```python
from build123d import *

# Parameters (mm, degrees)
F0_W         = 62.5
F0_H         = 36.5
F0_W_2       = 58.5
F0_H_2       = 31.5
F1_DEPTH     = 7
F3_DEPTH     = 1.5
F4_W         = 62.5
F4_H         = 36.5
F5_DEPTH     = 3
F7_DEPTH     = 2.5
F8_R         = 2.5
F9_T1_DEPTH  = 57.5
F9_T3_DEPTH  = 31.5
F9_T6_ANGLE  = 90
F9_T8_ANGLE  = 90
F9_T10_ANGLE = 90
F9_T12_ANGLE = 90
F10_W        = 1.25
F10_H        = 8.5
F11_DEPTH    = 2
F13_DEPTH    = 3


# Not quite as in the source:
# - a fillet or chamfer that OpenCascade refuses, or shapes differently, is made with other operations: its cross-section is extruded or revolved along the edge and cut away or added
# - a feature names something its author has since deleted; it is built from what else it names


with BuildPart() as f1:
    # F0 (on Top) → F1 (new body)
    with BuildSketch(Plane.XY):
        with Locations((0.5, 0.5)):
            Rectangle(F0_W, F0_H)
        with Locations((1, 0.5)):
            Rectangle(F0_W_2, F0_H_2, mode=Mode.SUBTRACT)
    extrude(amount=F1_DEPTH)

    # F2 (on face) → F3 (join)
    with BuildSketch(Plane.XY.offset(7)):
        Polygon((30.25, 16.25), (-28.25, 16.25), (-28.25, -15.25), (30.25, -15.25), (30.25, -6), (30.25, 7), align=None)
    extrude(amount=-F3_DEPTH)

    # F4 (on face) → F5 (join)
    with BuildSketch(Plane(origin=(0, 0, 0), x_dir=(1, 0, 0), z_dir=(0, 0, -1))):
        with Locations((0.5, -0.5)):
            Rectangle(F4_W, F4_H)
        Polygon((-29.5, -17.522141248), (-29.5, 16.5), (30.25, 16.5), (30.25, 15.25), (30.25, -16.25), (30.25, -17.522141248), align=None, mode=Mode.SUBTRACT)
    extrude(amount=F5_DEPTH)

    # F6 (on face) → F7 (cut)
    with BuildSketch(Plane.YZ.offset(-28.25)):
        with BuildLine():
            Line((4, 5.5), (-3, 5.5))
            ThreePointArc((-3, 5.5), (-3.5303300859, 5.2803300859), (-3.75, 4.75))
            Line((-3.75, 4.75), (-3.75, 3.5))
            ThreePointArc((-3.75, 3.5), (-3.1642135624, 2.0857864376), (-1.75, 1.5))
            Line((-1.75, 1.5), (2.75, 1.5))
            ThreePointArc((2.75, 1.5), (4.1642135624, 2.0857864376), (4.75, 3.5))
            Line((4.75, 3.5), (4.75, 4.75))
            ThreePointArc((4.75, 4.75), (4.5303300859, 5.2803300859), (4, 5.5))
        make_face()
    extrude(amount=-F7_DEPTH, mode=Mode.SUBTRACT)

    # F8
    f8_edges = [f1.edges().sort_by_distance(p)[0] for p in [
        (-30.75, 18.75, 2),
        (-30.75, -17.75, 2),
        (31.75, 18.75, 2),
        (31.75, -17.75, 2),
    ]]
    fillet(f8_edges, radius=F8_R)

    # F9: fillet of radius 2 on 8 edges, made by hand

    # F9_s2 → F9_t1 (cut)
    with BuildSketch(Plane.YZ.offset(-28.25)):
        with BuildLine():
            ThreePointArc((18.75, 5), (18.1642135624, 6.4142135624), (16.75, 7))
            Line((16.75, 7), (18.75, 7))
            Line((18.75, 7), (18.75, 5))
        make_face()
        with BuildLine():
            ThreePointArc((-15.75, 7), (-17.1642135624, 6.4142135624), (-17.75, 5))
            Line((-17.75, 5), (-17.75, 7))
            Line((-17.75, 7), (-15.75, 7))
        make_face()
    extrude(amount=F9_T1_DEPTH, mode=Mode.SUBTRACT)

    # F9_s4 → F9_t3 (cut)
    with BuildSketch(Plane.XZ.offset(-16.25)):
        with BuildLine():
            ThreePointArc((29.75, 7), (31.1642135624, 6.4142135624), (31.75, 5))
            Line((31.75, 5), (31.75, 7))
            Line((31.75, 7), (29.75, 7))
        make_face()
        with BuildLine():
            ThreePointArc((-28.75, 7), (-30.1642135624, 6.4142135624), (-30.75, 5))
            Line((-30.75, 5), (-30.75, 7))
            Line((-30.75, 7), (-28.75, 7))
        make_face()
    extrude(amount=F9_T3_DEPTH, mode=Mode.SUBTRACT)

    # F9_s5 → F9_t6 (revolve, cut)
    with BuildSketch(Plane.YZ.offset(29.25)):
        with BuildLine():
            ThreePointArc((16.75, 7), (18.1642135624, 6.4142135624), (18.75, 5))
            Line((18.75, 5), (18.75, 7))
            Line((18.75, 7), (16.75, 7))
        make_face()
    revolve(axis=Axis((29.25, 16.25, 7), (0, 0, -1)), revolution_arc=F9_T6_ANGLE, mode=Mode.SUBTRACT)

    # F9_s7 → F9_t8 (revolve, cut)
    with BuildSketch(Plane.YZ.offset(-28.25)):
        with BuildLine():
            ThreePointArc((16.75, 7), (18.1642135624, 6.4142135624), (18.75, 5))
            Line((18.75, 5), (18.75, 7))
            Line((18.75, 7), (16.75, 7))
        make_face()
    revolve(axis=Axis((-28.25, 16.25, 7), (0, 0, 1)), revolution_arc=F9_T8_ANGLE, mode=Mode.SUBTRACT)

    # F9_s9 → F9_t10 (revolve, cut)
    with BuildSketch(Plane.XZ.offset(15.25)):
        with BuildLine():
            ThreePointArc((29.75, 7), (31.1642135624, 6.4142135624), (31.75, 5))
            Line((31.75, 5), (31.75, 7))
            Line((31.75, 7), (29.75, 7))
        make_face()
    revolve(axis=Axis((29.25, -15.25, 7), (0, 0, -1)), revolution_arc=F9_T10_ANGLE, mode=Mode.SUBTRACT)

    # F9_s11 → F9_t12 (revolve, cut)
    with BuildSketch(Plane.XZ.offset(15.25)):
        with BuildLine():
            ThreePointArc((-28.75, 7), (-30.1642135624, 6.4142135624), (-30.75, 5))
            Line((-30.75, 5), (-30.75, 7))
            Line((-30.75, 7), (-28.75, 7))
        make_face()
    revolve(axis=Axis((-28.25, -15.25, 7), (0, 0, 1)), revolution_arc=F9_T12_ANGLE, mode=Mode.SUBTRACT)

    # F10 (on face) → F11 (cut)
    with BuildSketch(Plane(origin=(0, 0, 0), x_dir=(1, 0, 0), z_dir=(0, 0, -1))):
        with Locations((-28.875, -0.5)):
            Rectangle(F10_W, F10_H)
    extrude(amount=-F11_DEPTH, mode=Mode.SUBTRACT)

    # F12 (on face) → F13 (cut)
    with BuildSketch(Plane.XY.offset(7)):
        with BuildLine():
            ThreePointArc((22.6871086181, -10.5021475209), (24.4149310408, -5.3769082449), (25, 0))
            ThreePointArc((25, 0), (24.4149310408, 5.3769082449), (22.6871086181, 10.5021475209))
            Line((22.6871086181, 10.5021475209), (21.325882101, 9.8720186697))
            ThreePointArc((21.325882101, 9.8720186697), (22.9500351783, 5.0542937502), (23.5, 0))
            ThreePointArc((23.5, 0), (22.9500351783, -5.0542937502), (21.325882101, -9.8720186697))
            Line((21.325882101, -9.8720186697), (22.6871086181, -10.5021475209))
        make_face()
        with BuildLine():
            ThreePointArc((19.5109134115, -9.031846868), (20.9968406951, -4.6241410906), (21.5, 0))
            ThreePointArc((21.5, 0), (20.9968406951, 4.6241410906), (19.5109134115, 9.031846868))
            Line((19.5109134115, 9.031846868), (18.1496868945, 8.4017180168))
            ThreePointArc((18.1496868945, 8.4017180168), (19.5319448326, 4.3015265959), (20, 0))
            ThreePointArc((20, 0), (19.5319448326, -4.3015265959), (18.1496868945, -8.4017180168))
            Line((18.1496868945, -8.4017180168), (19.5109134115, -9.031846868))
        make_face()
        with BuildLine():
            ThreePointArc((16.334718205, -7.5615462151), (17.5787503494, -3.8713739363), (18, 0))
            ThreePointArc((18, 0), (17.5787503494, 3.8713739363), (16.334718205, 7.5615462151))
            Line((16.334718205, 7.5615462151), (14.9734916879, 6.9314173638))
            ThreePointArc((14.9734916879, 6.9314173638), (16.1138544869, 3.5487594416), (16.5, 0))
            ThreePointArc((16.5, 0), (16.1138544869, -3.5487594416), (14.9734916879, -6.9314173638))
            Line((14.9734916879, -6.9314173638), (16.334718205, -7.5615462151))
        make_face()
    extrude(amount=-F13_DEPTH, mode=Mode.SUBTRACT)


solid = f1.part
```
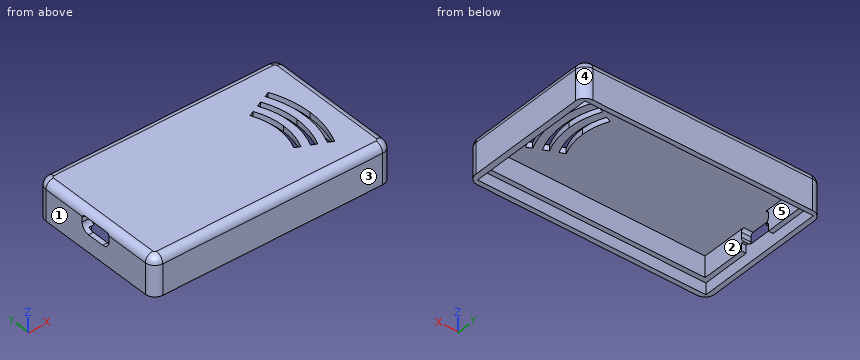
Here's how the part is built. I have some questions about the finished solid (model axes, mm). Face numbers are marked on the shaded views. A direction names the side the tool comes from. Coordinates: 2 decimals unless noted, no trailing zeros. Order: outer loops, then holes, each group sorted by start corner. A loop starts at its lowest first (then second) coordinate and runs counter-clockwise, first axis right, second up. Notation, with made-up numbers: (26, 54) -> (47, 54) arc R25 cw to (47, 87) -> close; hole circle Ø1 at (79.25, 11). An arc over 180 degrees is marked (long way). Return JSON: item names as keys, results as strings.
1) Thinking about a two-plate mould opening in Y: for the marked faces 3, 4 and 5, which applies, +Y half, -Y half, draft (parallel to the pull), parting line (faces both ways), or undercut?
Conclusion:
{"face 3": "-Y half", "face 4": "+Y half", "face 5": "undercut"}
2) On a 3-axis mill with a long thin cutter (end or side, diameter ignored), from which of +Z, -Z, +X, -X, +Y, -Y can I reach the whole of each face in a straight line? I mean the marked faces 1 and 2. Say none if no direction works.
Conclusion:
{"face 1": "+Z, -Z, -X, +Y, -Y", "face 2": "-Z"}
3) If we section it at B-B on x = 8: List the corners of the cut face in (y, z) for me.
Conclusion:
{"outline": "(-17.75, -3) -> (-16.5, -3) -> (-16.5, 0) -> (-15.25, 0) -> (-15.25, 5.5) -> (16.25, 5.5) -> (16.25, 0) -> (17.52, 0) -> (17.52, -3) -> (18.75, -3) -> (18.75, 5) arc R2 ccw to (16.75, 7) -> (-15.75, 7) arc R2 ccw to (-17.75, 5) -> close"}
4) If we section it at A-A on z = -0.75: List the corners of the cut face in (x, y) for me, plus the area to 3 significant figures.
Conclusion:
{"outline": "(-30.75, -15.25) arc R2.5 ccw to (-28.25, -17.75) -> (29.25, -17.75) arc R2.5 ccw to (31.75, -15.25) -> (31.75, 16.25) arc R2.5 ccw to (29.25, 18.75) -> (-28.25, 18.75) arc R2.5 ccw to (-30.75, 16.25) -> close; hole (-29.5, -16.5) -> (30.25, -16.5) -> (30.25, 17.52) -> (-29.5, 17.52) -> close", "area": "243 mm²"}
5) If I drill on probe 1 along X at (y, z) = (-3, 0.25); probe 2 along X at (y, z) = (-5, 4.5); probe 3 along Y at (x, z) = (1, 1.25), over which ranges is the centre line in solid material (lowest first)?
Conclusion:
{"probe 1": "x = -30.75 to -29.5, 30.25 to 31.75", "probe 2": "x = -30.75 to -28.25, 30.25 to 31.75", "probe 3": "y = -17.75 to -15.25, 16.25 to 18.75"}
6) I'm going to push flat-ended pins straight in: P1, Ø0.6, axis at x = -29, z = 1, coming from the +Y side; P2, Ø14, axis at x = -2.5, y = 13, coming from the -Z side; P3, Ø6, axis at x = 20.5, y = 2, coming from the -Z side. Where does each tip first touch, or does it pass through?
Conclusion:
{"P1": "stops at y = 18.71", "P2": "stops at z = -3", "P3": "stops at z = 5.5"}
7) If we section it at C-C on y = -13: List the corners of the cut face in (x, z) for me, plus the area to 3 significant figures.
Conclusion:
{"outline": "(-30.75, -3) -> (-29.5, -3) -> (-29.5, 0) -> (-28.25, 0) -> (-28.25, 5.5) -> (30.25, 5.5) -> (30.25, -3) -> (31.75, -3) -> (31.75, 5) arc R2 ccw to (29.75, 7) -> (-28.75, 7) arc R2 ccw to (-30.75, 5) -> close", "area": "122 mm²"}
